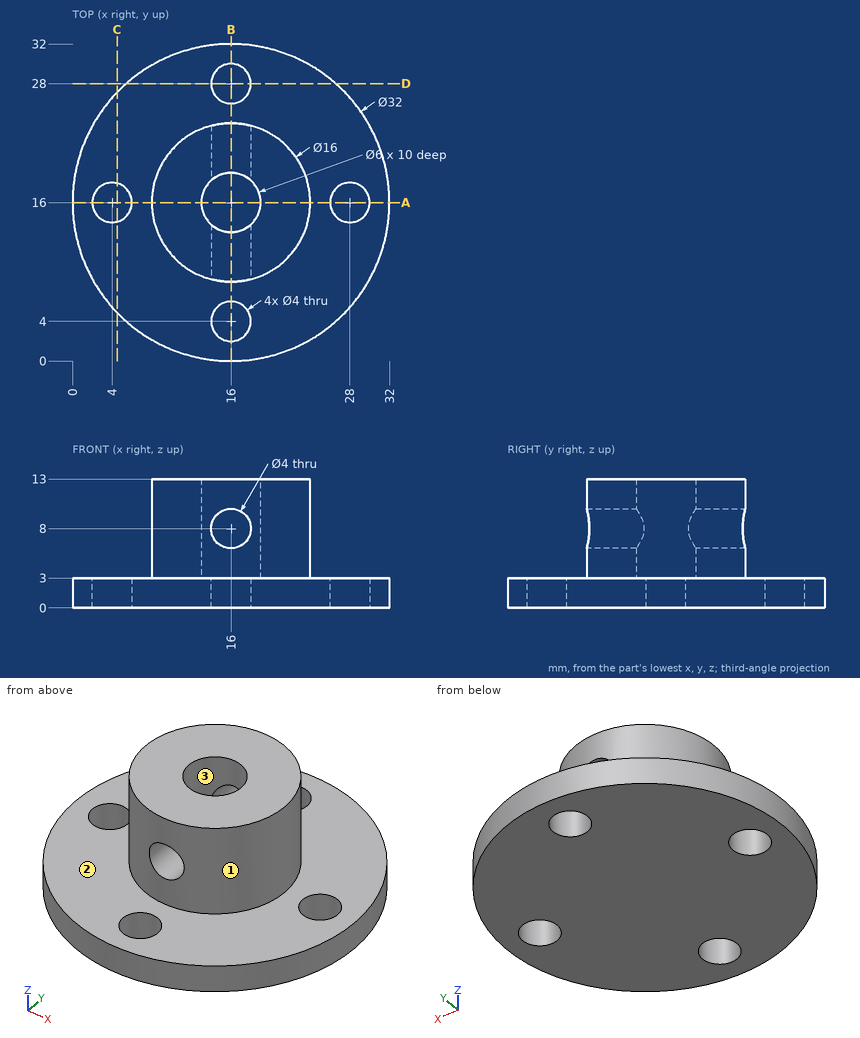
Drawing for the job (mm, zero at the part's lowest x, y, z). Round coordinates to 2 decimals unless told otherwise and drop trailing zeros. Loops run counter-clockwise (first coordinate to the right, second up) from the corner with the lowest first, then second, coordinate; pieces in that order, holes last. Notation, with made-up numbers: (39.5, -22.75) - (61.5, -22.75) arc R4 cw to (61.5, -18.75) - close; hole circle Ø1 at (49.25, 44.25). An arc over 180 degrees is marked (long way). Write each question's results on one line, items separated by ' | '.
(1) Mould opens along Y. For the marked faces 1, 2 and 3 say: released by +Y, released by -Y, zero draft, split by the parting line, or undercut.
Answer below:
face 1: split by the parting line | face 2: zero draft | face 3: undercut
(2) Saw through at B-B, the plane x = 16. List the corners of the cut face in (y, z).
Answer below:
outline: (0, 0) - (2, 0) - (2, 3) - (0, 3) - close; (6, 0) - (26, 0) - (26, 3) - (24, 3) - (24, 6) - (19, 6) - (19, 3) - (13, 3) - (13, 6) - (8, 6) - (8, 3) - (6, 3) - close; (8, 10) - (13, 10) - (13, 13) - (8, 13) - close; (19, 10) - (24, 10) - (24, 13) - (19, 13) - close; (30, 0) - (32, 0) - (32, 3) - (30, 3) - close
(3) Wall check: L1, parallel to Y at x = 16, z = 1.5; L2, parallel to Z at x = 16, y = 21; L3, parallel to Z at x = 29.5, y = 7.5. Give the ranges that are in metal, low to high.
Answer below:
L1: y = 0 to 2, 6 to 26, 30 to 32 | L2: z = 0 to 6, 10 to 13 | L3: z = 0 to 3
(4) Saw through at A-A, the plane y = 16. List the corners of the cut face in (x, z), then the cut area to 3 significant figures.
Answer below:
outline: (0, 0) - (2, 0) - (2, 3) - (0, 3) - close; (6, 0) - (26, 0) - (26, 3) - (24, 3) - (24, 13) - (19, 13) - (19, 3) - (13, 3) - (13, 13) - (8, 13) - (8, 3) - (6, 3) - close; (30, 0) - (32, 0) - (32, 3) - (30, 3) - close | area: 172 mm^2
(5) Saw through at C-C, the plane x = 4.5. List the corners of the cut face in (y, z), then the cut area to 3 significant figures.
Answer below:
outline: (4.88, 0) - (14.06, 0) - (14.06, 3) - (4.88, 3) - close; (17.94, 0) - (27.12, 0) - (27.12, 3) - (17.94, 3) - close | area: 55.1 mm^2
(6) Saw through at D-D, the plane y = 28. List the corners of the cut face in (x, z), then the cut area to 3 significant figures.
Answer below:
outline: (5.42, 0) - (14, 0) - (14, 3) - (5.42, 3) - close; (18, 0) - (26.58, 0) - (26.58, 3) - (18, 3) - close | area: 51.5 mm^2
(7) Pin check, flat tips, straight feed: pin 1 (1.5 mm diameter, centred on x = 28, y = 12, fed in from -Z); pin 2 (2 mm diameter, centred on y = 12.5, z = 11, fed in from -X); pin 3 (2.5 mm diameter, centred on x = 28, y = 16, fed in from -Z); pin 4 (3.5 mm diameter, centred on x = 16, y = 16, fed in from +Z). Stop position of each tip, or through.
Answer below:
pin 1: stops at z = 0 | pin 2: stops at x = 8.4 | pin 3: passes through | pin 4: stops at z = 3
